```python
from build123d import *

# Parameters (mm, degrees)
SKETCH_1_R      = 28.5
EXTRUDE_1_DEPTH = 30


with BuildPart() as part:
    # 草图1 → 凸台-拉伸1 (new body)
    with BuildSketch(Plane(origin=(0, 0, 0), x_dir=(1, 0, 0), z_dir=(0, 1, 0))):
        with BuildLine():
            Line((0, -38.5), (300, -38.5))
            ThreePointArc((300, -38.5), (338.5, 0), (300, 38.5))
            Line((300, 38.5), (0, 38.5))
            ThreePointArc((0, 38.5), (-38.5, 0), (0, -38.5))
        make_face()
        with Locations(Location((0, 0, 0), (0, 0, 270))):
            Circle(SKETCH_1_R, mode=Mode.SUBTRACT)
        with Locations(Location((300, 0, 0), (0, 0, 90))):
            Circle(SKETCH_1_R, mode=Mode.SUBTRACT)
        with BuildLine():
            Line((28.354893758, -28.5), (271.645106242, -28.5))
            ThreePointArc((271.645106242, -28.5), (272.566030379, -27.889741881), (272.362951654, -26.803797468))
            ThreePointArc((272.362951654, -26.803797468), (261.5, 0), (272.362951654, 26.803797468))
            ThreePointArc((272.362951654, 26.803797468), (272.566030379, 27.889741881), (271.645106242, 28.5))
            Line((271.645106242, 28.5), (28.354893758, 28.5))
            ThreePointArc((28.354893758, 28.5), (27.433969621, 27.889741881), (27.637048346, 26.803797468))
            ThreePointArc((27.637048346, 26.803797468), (38.5, 0), (27.637048346, -26.803797468))
            ThreePointArc((27.637048346, -26.803797468), (27.433969621, -27.889741881), (28.354893758, -28.5))
        make_face(mode=Mode.SUBTRACT)
    extrude(amount=EXTRUDE_1_DEPTH)


solid = part.part
```
Work out the finished part from the listing and answer in its coordinate system (mm). A direction names the side the tool comes from. Give positions to 0.01 mm unless a question says otherwise; leave off trailing zeros. Loops run counter-clockwise (first coordinate to the right, second up) from the corner with the lowest first, then second, coordinate; pieces in that order, holes last. Notation, with made-up numbers: M 44.25,84 L 51.25,84 A7 ccw 51.25,96 Z; hole C -19.5,44 d6. An arc over 180 degrees is marked long. One line per item, written item: value. Start each with the question number.
1. Which of the six approach directions +Z, -Z, +X, -X, +Y, -Y give full straight-line access (tool end or side, diameter ignored) to faces 1 (the face through (38.498, 14.79, -0.415)), 2 (the face through (135, 30, -29))?
2. Find section A-A (x = 144.5). Give the vertices of the cut face in (y, z).
3. Find section D-D (x = -4.5). Give the vertices of the cut face in (y, z).
4. Find section B-B (z = 0). Give the vertices of the cut face in (x, y).
5. Determine the mould class of faces 3 (the face through (152, 15, -38.5)), 4 (the face through (148, 15, 28.5)), 5 (the face through (135, 0, -29)) for opening direction Z: released by +Z, released by -Z, zero draft, split by the parting line, or undercut.
6. Find the intervals of material crossed by probe 1 along X at (y, z) = (11.5, -0.5); probe 2 along Z at (x, y) = (152, 7); probe 3 along Z at (x, y) = (2, 7.5), in increasing order.
7. Find section C-C (y = 12.5). Give the vertices of the cut face in (x, z).
8. This flat-tipped pin is pushed along its axis until it touches: P1, Ø6, axis at y = 5.5, z = -30.5, coming from the +X side. Where does it stop, or does it pass through?
Reported:
1. face 1: +Y, -Y
1. face 2: +Z, -Z, +X, -X, +Y
2. outline: M 0,-38.5 L 30,-38.5 L 30,-28.5 L 0,-28.5 Z; M 0,28.5 L 30,28.5 L 30,38.5 L 0,38.5 Z
3. outline: M 0,-38.24 L 30,-38.24 L 30,-28.14 L 0,-28.14 Z; M 0,28.14 L 30,28.14 L 30,38.24 L 0,38.24 Z
4. outline: M -38.5,0 L -28.5,0 L -28.5,30 L -38.5,30 Z; M 28.5,0 L 38.5,0 L 38.5,30 L 28.5,30 Z; M 261.5,0 L 271.5,0 L 271.5,30 L 261.5,30 Z; M 328.5,0 L 338.5,0 L 338.5,30 L 328.5,30 Z
5. face 3: released by -Z
5. face 4: undercut
5. face 5: zero draft
6. probe 1: x = -38.5 to -28.5, 28.5 to 38.5, 261.5 to 271.5, 328.5 to 338.5
6. probe 2: z = -38.5 to -28.5, 28.5 to 38.5
6. probe 3: z = -38.5 to -28.43, 28.43 to 38.5
7. outline: M 0,-38.5 L 300,-38.5 A38.5 ccw 300,38.5 L 0,38.5 A38.5 ccw Z; hole C 0,0 d57; hole M 27.64,-26.8 A1 ccw 28.35,-28.5 L 271.65,-28.5 A1 ccw 272.36,-26.8 A38.5 cw 272.36,26.8 A1 ccw 271.65,28.5 L 28.35,28.5 A1 ccw 27.64,26.8 A38.5 cw Z; hole C 300,0 d57
8. P1: stops at x = 326.94
